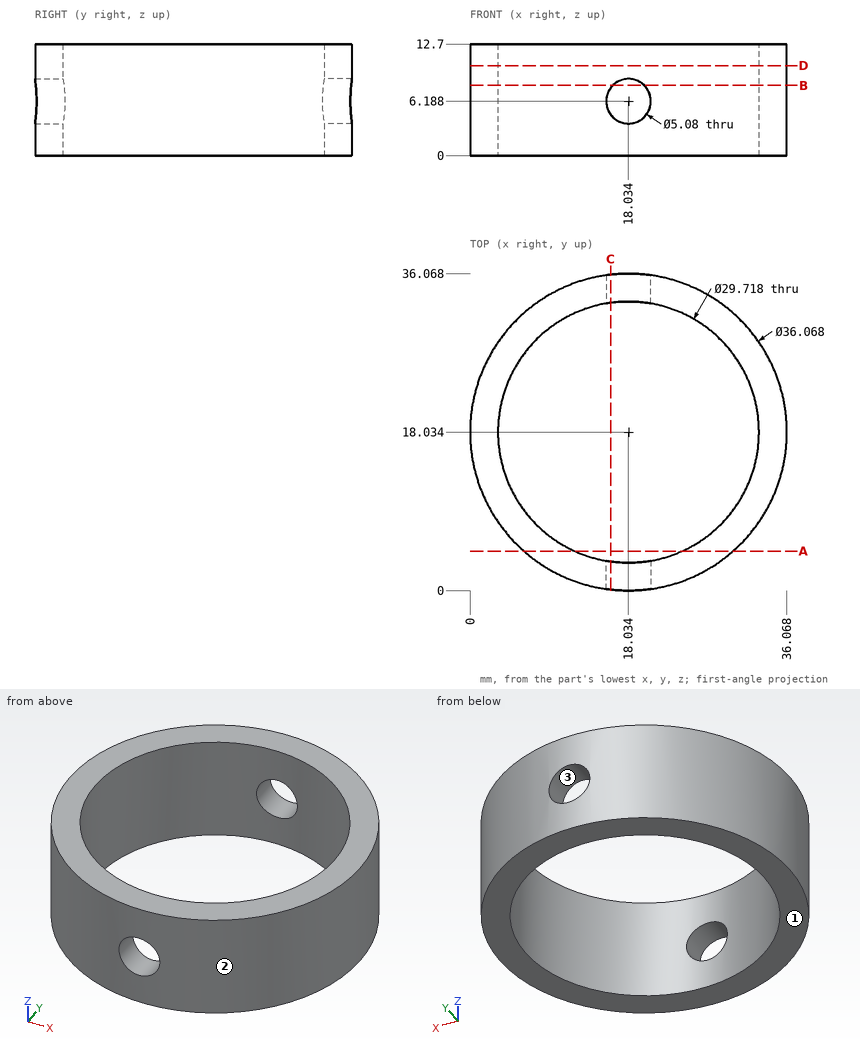
Verification items for this drawing (mm, ordinates from the low corner). Give positions to 0.01 mm unless a question says otherwise; leave off trailing zeros. Write each loop counter-clockwise with the first axis right and the second up, starting at its lowest first coordinate (ties: lowest second). Pieces come first, ordered by that corner, then holes. Notation, with made-up numbers: (82.5, 80.25) -> (139.5, 80.25) arc R32 cw to (139.5, 106.25) -> close; hole circle Ø2 at (61.5, -37). An arc over 180 degrees is marked (long way). Use CSV: the item, a comma, the result in double quotes. Start each with the question number.
Q1. Cross-section at A-A on y = 4.5. Enter the section's corners in (x, z) (1 decimal), and give its area (3 significant figures).
Q2. Cross-section at B-B on z = 8. Enter the section's corners in (x, y).
Q3. Scan lines: line 1 along Y through (x, z) = (11, 0.5) (1 decimal); line 2 along Y through (x, z) = (14, 11.5) (1 decimal); line 3 along X through (y, z) = (23, 5.25). Record each from-to range of solid material in increasing order.
Q4. Cross-section at D-D on z = 10.25. Enter the section's corners in (x, y), and give its area (3 significant figures).
Q5. Depth check by flat-ended pin: P1, Ø3, axis at y = 28, z = 3, coming from the -X side. Enter the tip coordinate at first touch or a pass-through.
Q6. Release check for a two-part mould opening along X. For the marked faces 1, 2 and 3 record: +X half, -X half, draft (parallel to the pull), parting line (faces both ways), or undercut.
Q7. Cross-section at C-C on x = 16. Enter the section's corners in (y, z) (1 decimal), and give its area (3 significant figures).
Working result:
1,outline,"(6.1, 0) -> (11.9, 0) -> (11.9, 12.7) -> (6.1, 12.7) -> close; (24.2, 0) -> (30, 0) -> (30, 12.7) -> (24.2, 12.7) -> close"
1,area,"147 mm^2"
2,outline,"(16.25, 0.09) -> (16.25, 3.28) arc R14.86 cw to (16.25, 32.79) -> (16.25, 35.98) arc R18.03 ccw to start; (19.81, 0.09) arc R18.03 ccw to (19.81, 35.98) -> (19.81, 32.79) arc R14.86 cw to (19.81, 3.28) -> close"
3,line 1,"y = 1.4 to 4.9, 31.1 to 34.6"
3,line 2,"y = 0.5 to 3.7, 32.3 to 35.6"
3,line 3,"x = 0.7 to 4.03, 32.04 to 35.37"
4,outline,"circle Ø36.07 at (18.03, 18.03); hole circle Ø29.72 at (18.03, 18.03)"
4,area,"328 mm^2"
5,P1,"stops at x = 2.11"
6,face 1,"draft"
6,face 2,"parting line"
6,face 3,"undercut"
7,outline,"(0.1, 0) -> (3.3, 0) -> (3.3, 4.7) -> (0.1, 4.7) -> close; (0.1, 7.7) -> (3.3, 7.7) -> (3.3, 12.7) -> (0.1, 12.7) -> close; (32.8, 0) -> (36, 0) -> (36, 4.7) -> (32.8, 4.7) -> close; (32.8, 7.7) -> (36, 7.7) -> (36, 12.7) -> (32.8, 12.7) -> close"
7,area,"61.8 mm^2"
